For this review, take the finished solid that the model builds, in its own axes (mm). Face numbers are marked on the shaded views. A direction names the side the tool comes from. Round coordinates to 2 decimals unless told otherwise and drop trailing zeros. Order: outer loops, then holes, each group sorted by start corner. A loop starts at its lowest first (then second) coordinate and runs counter-clockwise, first axis right, second up.
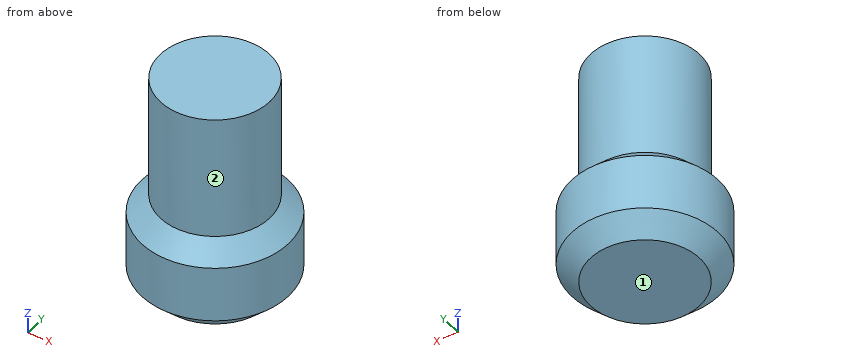
from build123d import *

# Parameters (mm, degrees)
F1_DEPTH = 25.4
F2_SIZE  = 5.08
F3_DEPTH = 33.782


with BuildPart() as f1:
    # F0 (on Top) → F1 (new body)
    with BuildSketch(Plane.XY):
        with BuildLine():
            ThreePointArc((-13.5880994109, 14.6109584599), (-7.9685359746, -18.2925937783), (19.9528582593, 0))
            ThreePointArc((19.9528582593, 0), (7.9685359746, 18.2925937783), (-13.5880994109, 14.6109584599))
        make_face()
    extrude(amount=F1_DEPTH)

    # F2
    f2_edges = [f1.edges().sort_by_distance(p)[0] for p in [
        (-19.952858, 0, 0),
        (19.952858, 0, 12.7),
        (-19.952858, 0, 25.4),
    ]]
    chamfer(f2_edges, length=F2_SIZE)

    # F3 (add): a face of the model
    f3_faces = [f1.faces().sort_by_distance(p)[0] for p in [
        (0, 0, 25.4),
    ]]
    extrude(f3_faces, amount=F3_DEPTH)


solid = f1.part
(1) Clearance check with flat-ended pins moving along their axes: P1, Ø1, axis at x = 12.5, z = 17, coming from the +Y side; P2, Ø2, axis at x = -4, z = 50.5, coming from the -Y side; P3, Ø5, axis at x = 3, z = 32, coming from the -Y side. State where each tip first meets the part, or that it passes through.
(2) Add section C-C on z = 43.5. Give the boundary of the cut face in (x, y).
(3) Tool access review of the marked faces 1 and 2: name each direction out of +Z, -Z, +X, -X, +Y, -Y from which nothing blocks a thin tool from reaching the whole face with its end or side.
(4) Add section A-A on x = 0. Give the boundary of the cut face in (y, z).
(5) Wall thickness on L1, parallel to Z at x = -13.5, y = 9; L2, parallel to X at y = -13, z = 48; L3, parallel to X at y = 12, z = 37: over which ranges is each line inside the solid? List them lowest first.
(6) Add section D-D on z = 6. Give the boundary of the cut face in (x, y), plus the area to 3 significant figures.
Here are the results:
1. P1: stops at y = 15.94
1. P2: stops at y = -14.57
1. P3: stops at y = -14.86
2. outline: circle Ø29.75 at (0, 0)
3. face 1: -Z, +X, -X, +Y, -Y
3. face 2: +Z
4. outline: (-19.95, 5.08) - (-14.87, 0) - (14.87, 0) - (19.95, 5.08) - (19.95, 20.32) - (14.87, 25.4) - (14.87, 59.18) - (-14.87, 59.18) - (-14.87, 25.4) - (-19.95, 20.32) - close
5. L1: z = 1.35 to 24.05
5. L2: x = -7.23 to 7.23
5. L3: x = -8.79 to 8.79
6. outline: circle Ø39.91 at (0, 0)
6. area: 1,250 mm2
